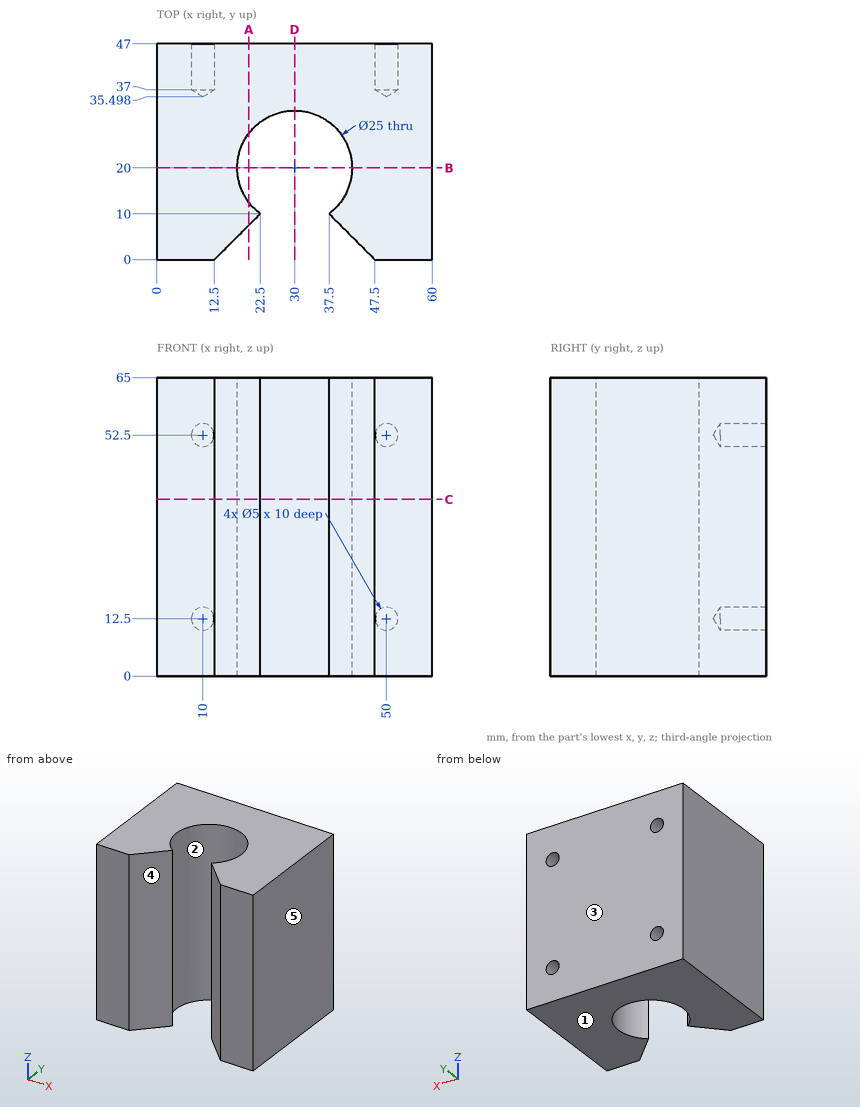
Print and shaded views of the part. All mm, measured from the part's lowest x, y and z. A direction names the side the tool comes from. Round coordinates to 2 decimals unless told otherwise and drop trailing zeros. Write each loop counter-clockwise with the first axis right and the second up, starting at its lowest first coordinate (ties: lowest second). Pieces come first, ordered by that corner, then holes. Notation, with made-up numbers: (54.25, 84.5) - (80.25, 84.5) arc R23 cw to (80.25, 95.5) - close; hole circle Ø8 at (68, 58). An arc over 180 degrees is marked (long way). Use CSV: the item, a comma, the result in double quotes. Start each with the question number.
Item 1: Band-saw the part on D-D (x = 30). Write the cut outline in (y, z).
Item 2: Drill centre lines: L1, parallel to X at y = 39.25, z = 12.5; L2, parallel to Z at x = 50, y = 41; L3, parallel to X at y = 40, z = 12. Where is each one in solid material? Low to high. Write a range as [from, to].
Item 3: Two-plate mould, pull along Y, no slides. Class the marked faces 1, 2 and 3: released by +Y, released by -Y, zero draft, split by the parting line, or undercut.
Item 4: Pin check, flat tip, straight feed: P1, Ø4, axis at x = 50, z = 52.5, coming from the +Y side. Stop position of the tip, or through.
Item 5: Band-saw the part on C-C (z = 38.5). Write the cut outline in (x, y).
Item 6: Band-saw the part on A-A (x = 20). Write the cut outline in (y, z), and give its area (3 significant figures).
Item 7: Tool access for the marked faces 4 and 5: list every direction of +Z, -Z, +X, -X, +Y, -Y with a clear straight run to the whole face (end or side of a thin tool).
Item 8: Band-saw the part on B-B (y = 20). Write the cut outline in (x, z).
Checked values:
1,outline,"(32.5, 0) - (47, 0) - (47, 65) - (32.5, 65) - close"
2,L1,"x = [0, 7.5], [12.5, 47.5], [52.5, 60]"
2,L2,"z = [0, 10], [15, 50], [55, 65]"
2,L3,"x = [0, 7.55], [12.45, 47.55], [52.45, 60]"
3,face 1,"zero draft"
3,face 2,"undercut"
3,face 3,"released by +Y"
4,P1,"stops at y = 36.7"
5,outline,"(0, 0) - (12.5, 0) - (22.5, 10) arc R12.5 cw (long way) to (37.5, 10) - (47.5, 0) - (60, 0) - (60, 47) - (0, 47) - close"
6,outline,"(7.5, 0) - (12.5, 0) - (12.5, 65) - (7.5, 65) - close; (27.5, 0) - (47, 0) - (47, 65) - (27.5, 65) - close"
6,area,"1,590 mm²"
7,face 4,"+Z, -Z, -Y"
7,face 5,"+Z, -Z, +X, +Y, -Y"
8,outline,"(0, 0) - (17.5, 0) - (17.5, 65) - (0, 65) - close; (42.5, 0) - (60, 0) - (60, 65) - (42.5, 65) - close"
